The listing builds one solid part. Answer for the finished solid, in the listing's coordinates (mm). A direction names the side the tool comes from. Give positions to 0.01 mm unless a question says otherwise; leave off trailing zeros. Order: outer loops, then holes, each group sorted by start corner. A loop starts at its lowest first (then second) coordinate and runs counter-clockwise, first axis right, second up. Notation, with made-up numbers: (-21.5, -15.5) - (-4.5, -15.5) arc R27 ccw to (-4.5, 6.5) - close; hole circle Ø8 at (74.25, 44). An arc over 180 degrees is marked (long way). Use a Markdown table: item, result. Add a question column.
1) Find section A-A, the plane z = 30. Determine the outline of the cut face in (x, y).
2) Flat-ended cylindrical pins translate along their axes: pin 1 (13 mm diameter, centred on x = -23.5, z = 99.5, fed in from -Y); pin 2 (1.2 mm diameter, centred on x = 10.5, y = -61, fed in from -Z); pin 3 (1.5 mm diameter, centred on y = -62, z = 52.5, fed in from +X); pin 4 (5 mm diameter, centred on y = -60, z = 45, fed in from -X). Find the tip coordinate at first contact, or state that the pin passes through.
3) Find section B-B, the plane x = 27.5. Determine the outline of the cut face in (y, z).
4) Straight lines are drawn through the part: line 1 (Z direction, x = 27.5, y = -67.3); line 2 (Z direction, x = -5, y = -58.75); line 3 (X direction, y = -59.75, z = 101). For each, find the intervals that lie inside material, in ascending order.
5) The mould has two halves that part along Z. Classify faces 1 (the face through (-1, -66, -22.5)), 2 (the face through (0, -61, 107)), 3 (the face through (-28, -67, -12)): released by +Z, released by -Z, zero draft, split by the parting line, or undercut.
6) Find section C-C, the plane y = -60.75. Determine the outline of the cut face in (x, z), plus the area to 3 significant figures.
7) Find section D-D, the plane z = -12.5. Determine the outline of the cut face in (x, y), plus the area to 3 significant figures.
8) For faces 4 (the face through (-28, -67, 103)), 5 (the face through (0, -61, -17)), 6 (the face through (32, -61, 44)), determine the directions among +Z, -Z, +X, -X, +Y, -Y from which every point of the face is accessible in a straight line to the end or side of a thin tool.
from build123d import *

# Parameters (mm, degrees)
SKETCH032_W     = 64
SKETCH032_H     = 124
PAD019_DEPTH    = 5
SKETCH033_W     = 75
SKETCH033_H     = 135
PAD020_DEPTH    = 5
FILLET001_R     = 1
SKETCH034_R     = 8.1
POCKET002_DEPTH = 1


with BuildPart() as part:
    # Sketch032 → Pad019 (new body)
    with BuildSketch(Plane.XZ):
        with Locations((0, 45)):
            Rectangle(SKETCH032_W, SKETCH032_H)
    extrude(amount=-PAD019_DEPTH)

    # Sketch033 → Pad020 (join)
    with BuildSketch(Plane.XZ):
        with Locations((0, 45)):
            Rectangle(SKETCH033_W, SKETCH033_H)
    extrude(amount=PAD020_DEPTH)

    # Fillet001
    fillet001_edges = [part.edges().sort_by_distance(p)[0] for p in [
        (0, 0, -22.5),
        (-37.5, 0, 45),
        (37.5, 0, 45),
        (32, 5, 45),
        (0, 5, -17),
        (0, 0, 112.5),
        (0, 5, 107),
        (-32, 5, 45),
    ]]
    fillet(fillet001_edges, radius=FILLET001_R)

    # Sketch034 (on Face19 of Fillet001) → Pocket002 (cut)
    with BuildSketch(Plane.XZ.offset(5)):
        with Locations((-27.5, 102.5)):
            Circle(SKETCH034_R)
        with Locations((27.5, 102.5)):
            Circle(SKETCH034_R)
        with Locations((-27.5, -12.5)):
            Circle(SKETCH034_R)
        with Locations((27.5, -12.5)):
            Circle(SKETCH034_R)
    extrude(amount=-POCKET002_DEPTH, mode=Mode.SUBTRACT)


with BuildPart() as part_1:
    # Body014 placement: moved
    add(part.part.moved(Location((0, -63, 0))))


solid = part_1.part
The answers:
| question | item | result |
|---|---|---|
| 1 | outline | (-37.5, -68) - (37.5, -68) - (37.5, -64) arc R1 ccw to (36.5, -63) - (32, -63) - (32, -59) arc R1 ccw to (31, -58) - (-31, -58) arc R1 ccw to (-32, -59) - (-32, -63) - (-36.5, -63) arc R1 ccw to (-37.5, -64) - close |
| 2 | pin 1 | y = -68 |
| 2 | pin 2 | z = -17 |
| 2 | pin 3 | x = 32 |
| 2 | pin 4 | x = -32 |
| 3 | outline | (-68, -22.5) - (-64, -22.5) arc R1 ccw to (-63, -21.5) - (-63, -17) - (-59, -17) arc R1 ccw to (-58, -16) - (-58, 106) arc R1 ccw to (-59, 107) - (-63, 107) - (-63, 111.5) arc R1 ccw to (-64, 112.5) - (-68, 112.5) - (-68, 110.6) - (-67, 110.6) - (-67, 94.4) - (-68, 94.4) - (-68, -4.4) - (-67, -4.4) - (-67, -20.6) - (-68, -20.6) - close |
| 4 | line 1 | -22.5 to -20.6, -4.4 to 94.4, 110.6 to 112.5 |
| 4 | line 2 | -16.97 to 106.97 |
| 4 | line 3 | -32 to 32 |
| 5 | face 1 | released by -Z |
| 5 | face 2 | released by +Z |
| 5 | face 3 | undercut |
| 6 | outline | (-32, -17) - (32, -17) - (32, 107) - (-32, 107) - close |
| 6 | area | 7,940 mm2 |
| 7 | outline | (-37.5, -68) - (-35.6, -68) - (-35.6, -67) - (-19.4, -67) - (-19.4, -68) - (19.4, -68) - (19.4, -67) - (35.6, -67) - (35.6, -68) - (37.5, -68) - (37.5, -64) arc R1 ccw to (36.5, -63) - (32, -63) - (32, -59) arc R1 ccw to (31, -58) - (-31, -58) arc R1 ccw to (-32, -59) - (-32, -63) - (-36.5, -63) arc R1 ccw to (-37.5, -64) - close |
| 7 | area | 662 mm2 |
| 8 | face 4 | -Y |
| 8 | face 5 | -Z, +X, -X, +Y |
| 8 | face 6 | +Z, -Z, +X, +Y |
